Input: part model. Units: mm. Frame: model coordinates. Face numbers are marked on the shaded views. A direction names the side the tool comes from. Coordinates: 2 decimals unless noted, no trailing zeros. Loops run counter-clockwise (first coordinate to the right, second up) from the corner with the lowest first, then second, coordinate; pieces in that order, holes last. Notation, with made-up numbers: (72, -26) - (110, -26) arc R25 ccw to (110, -9) - close; hole circle Ø3 at (66, 1.5). An arc over 180 degrees is marked (long way). Use one line per item in the form item = value.
from build123d import *

# Parameters (mm, degrees)
SKETCH2_W           = 70
SKETCH2_H           = 90
BOSS_EXTRUDE1_DEPTH = 1
SKETCH3_W           = 28
SKETCH3_H           = 22
BOSS_EXTRUDE2_DEPTH = 16
SKETCH4_W           = 30
SKETCH4_H           = 52
BOSS_EXTRUDE3_DEPTH = 15


with BuildPart() as part:
    # Sketch2 → Boss-Extrude1 (new body)
    with BuildSketch(Plane.XY):
        Rectangle(SKETCH2_W, SKETCH2_H)
    extrude(amount=BOSS_EXTRUDE1_DEPTH)

    # Sketch3 → Boss-Extrude2 (add)
    with BuildSketch(Plane.XY.offset(1)):
        with Locations((21, 26)):
            Rectangle(SKETCH3_W, SKETCH3_H)
    extrude(amount=BOSS_EXTRUDE2_DEPTH)

    # Sketch4 → Boss-Extrude3 (add)
    with BuildSketch(Plane.XY.offset(1)):
        with Locations((-20, -14)):
            Rectangle(SKETCH4_W, SKETCH4_H)
    extrude(amount=BOSS_EXTRUDE3_DEPTH)


solid = part.part
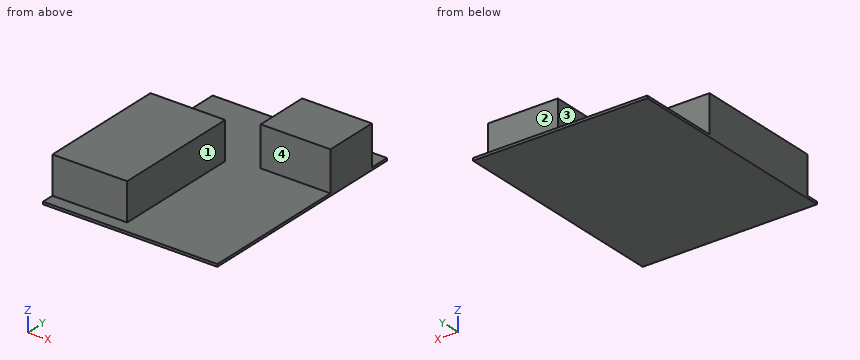
Q1. Cut plane D-D, the plane x = 17. Return loops of the section in (y, z), then the cut area to 3 significant figures.
Check values:
outline = (-45, 0) - (45, 0) - (45, 1) - (37, 1) - (37, 17) - (15, 17) - (15, 1) - (-45, 1) - close
area = 442 mm²
Q2. Cut plane B-B, the plane x = -14. Return loops of the section in (y, z).
Check values:
outline = (-45, 0) - (45, 0) - (45, 1) - (12, 1) - (12, 16) - (-40, 16) - (-40, 1) - (-45, 1) - close
Q3. Cut plane C-C, the plane y = -0.5. Return loops of the section in (x, z).
Check values:
outline = (-35, 0) - (35, 0) - (35, 1) - (-5, 1) - (-5, 16) - (-35, 16) - close
Q4. Set-up query: the marked faces 1, 2, 3 and 4. Return all of +Z, -Z, +X, -X, +Y, -Y with unobstructed straight access to the full face (end or side cutting, diameter ignored); none if empty.
Check values:
face_1 = +Z, +X, +Y, -Y
face_2 = +Z, +X, -X, +Y
face_3 = +Z, -X, +Y, -Y
face_4 = +Z, +X, -X, -Y
Q5. Ray query, line 1 along Y through (x, z) = (20, 2); line 2 along Y through (x, z) = (-31, 8.25); line 3 along X through (y, z) = (25.5, 10). Return the intervals inside material, ascending. Write a range as [from, to].
Check values:
line_1 = [15, 37]
line_2 = [-40, 12]
line_3 = [7, 35]
Q6. First-contact query: P1, Ø3, axis at y = -28, z = 13.5, coming from the +X side; P2, Ø4, axis at x = -6, z = 5, coming from the +Y side; P3, Ø12, axis at x = 22.5, y = 1, coming from the +Z side. Flat tips, straight axial feed; report the tip coordinate or a pass-through.
Check values:
P1 = -5
P2 = 12
P3 = 1
Q7. Cut plane A-A, the plane z = 11. Return loops of the section in (x, y), then the cut area to 3 significant figures.
Check values:
outline = (-35, -40) - (-5, -40) - (-5, 12) - (-35, 12) - close; (7, 15) - (35, 15) - (35, 37) - (7, 37) - close
area = 2,180 mm²
